Here's the drawing with two shaded views (mm, measured from the low corner). I have some questions. A direction names the side the tool comes from. Round coordinates to 2 decimals unless told otherwise and drop trailing zeros. Loops run counter-clockwise (first coordinate to the right, second up) from the corner with the lowest first, then second, coordinate; pieces in that order, holes last. Notation, with made-up numbers: M 49,-30.5 L 97,-30.5 A33 cw 97,2.5 Z; hole C -19.5,71.25 d4. An arc over 180 degrees is marked long. Answer as CSV lines item,"result".
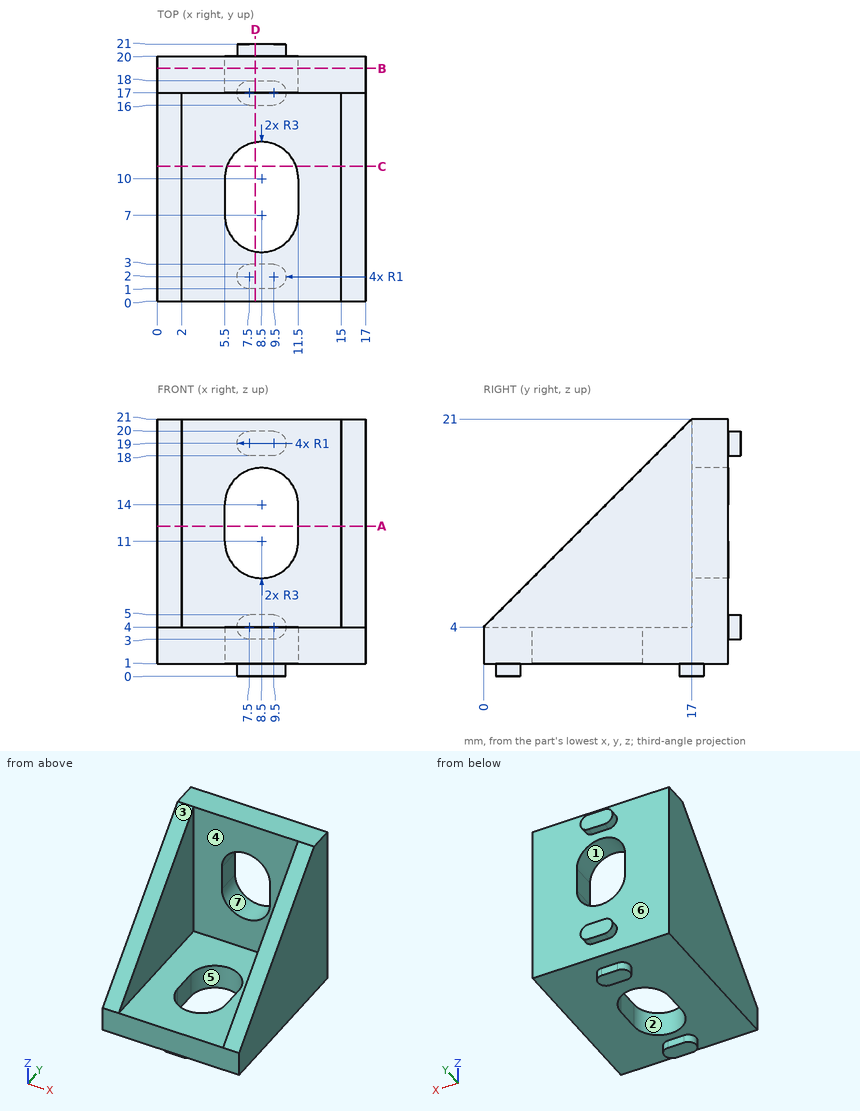
1. For P1, Ø0.9, axis at y = 19, z = 13, coming from the -X side; P2, Ø0.8, axis at x = 8, y = 20.5, coming from the -Z side; P3, Ø1.1, axis at x = 9, z = 0.5, coming from the +Y side; P4, Ø6.5, axis at x = 7, z = 9.5, coming from the -Y side, each with a flat end and sliding along its axis, tell me the tip position at first contact or that it passes through.
Evaluation:
P1,"stops at x = 0"
P2,"stops at z = 3"
P3,"stops at y = 20"
P4,"stops at y = 17"
2. I want a section at B-B, the plane y = 19. Please give me the cut outline in (x, z), and give its area (3 significant figures).
Evaluation:
outline,"M 0,1 L 17,1 L 17,21 L 0,21 Z; hole M 5.5,11 A3 ccw 11.5,11 L 11.5,14 A3 ccw 5.5,14 Z"
area,"294 mm²"
3. I want a section at D-D, the plane x = 8. Count the separate pieces of the cut face and the enclosed holes in it, and give its area (3 significant figures).
Evaluation:
separate pieces,"3"
enclosed holes,"0"
area,"65.5 mm²"
4. If I drill on line 1 (X direction, y = 8.5, z = 2.25); line 2 (X direction, y = 16.75, z = 9.5); line 3 (Y direction, x = 2.25, z = 10), over which ranges is the centre line in solid material (lowest first)? Write a range as [from, to].
Evaluation:
line 1,"x = [0, 5.5], [11.5, 17]"
line 2,"x = [0, 2], [15, 17]"
line 3,"y = [17, 20]"
5. I want a section at C-C, the plane y = 11. Please give me the cut outline in (x, z), and give its area (3 significant figures).
Evaluation:
outline,"M 0,1 L 5.67,1 L 5.67,4 L 2,4 L 2,15 L 0,15 Z; M 11.33,1 L 17,1 L 17,15 L 15,15 L 15,4 L 11.33,4 Z"
area,"78.0 mm²"
6. Which directions (+Z, -Z, +X, -X, +Y, -Y) give clear straight access to the entire face, cutting with the end or side of a thin tool? Please do the marked faces 1, 2, 3 and 4.
Evaluation:
face 1,"+Y, -Y"
face 2,"+Z, -Z"
face 3,"+Z, +X, -X, -Y"
face 4,"+Z, -Y"
7. We'd pull the mould along Y, two halves only. Please class the marked faces 5, 6 and 7: pulls with the +Y half, pulls with the -Y half, needs draft (parallel to the pull), parting line crosses it, or undercut.
Evaluation:
face 5,"undercut"
face 6,"pulls with the +Y half"
face 7,"needs draft"
8. I want a section at A-A, the plane z = 12.25. Please give me the cut outline in (x, y).
Evaluation:
outline,"M 0,8.25 L 2,8.25 L 2,17 L 5.5,17 L 5.5,20 L 0,20 Z; M 11.5,17 L 15,17 L 15,8.25 L 17,8.25 L 17,20 L 11.5,20 Z"
